```python
from build123d import *

# Parameters (mm, degrees)
SKETCH1_W                        = 39
SKETCH1_H                        = 37
BOSS_EXTRUDE1_DEPTH              = 6.5
SKETCH2_W                        = 30.2
SKETCH2_H                        = 4
CUT_EXTRUDE1_DEPTH               = 38
F_10_0_10_DIAMETER_HOLE1_D       = 10
F_10_0_10_DIAMETER_HOLE1_DEPTH   = 2.5
F_2_05_2_05_DIAMETER_HOLE1_D     = 2.05
F_2_05_2_05_DIAMETER_HOLE1_DEPTH = 6.5
F_2_05_2_05_DIAMETER_HOLE2_D     = 2.05
F_2_05_2_05_DIAMETER_HOLE2_DEPTH = 6.5
F_2_05_2_05_DIAMETER_HOLE3_D     = 2.05
F_2_05_2_05_DIAMETER_HOLE3_DEPTH = 6.5
CHAMFER1_SIZE                    = 0.25625
CHAMFER2_SIZE2                   = 0.199948225
CHAMFER2_SIZE                    = 0.199946154
SKETCH11_R                       = 1.28125
BOSS_EXTRUDE3_DEPTH              = 2.5
SKETCH12_R                       = 1.175
CUT_EXTRUDE2_DEPTH               = 7.5


with BuildPart() as part:
    # Sketch1 → Boss-Extrude1 (new body)
    with BuildSketch(Plane.XY.offset(-17)):
        with Locations((0, -3.5)):
            Rectangle(SKETCH1_W, SKETCH1_H)
    extrude(amount=-BOSS_EXTRUDE1_DEPTH)

    # Sketch2 → Cut-Extrude1 (cut, through all)
    with BuildSketch(Plane.XZ.offset(22)):
        with Locations((0, -19)):
            Rectangle(SKETCH2_W, SKETCH2_H)
    extrude(amount=-CUT_EXTRUDE1_DEPTH, mode=Mode.SUBTRACT)

    # Ø10.0 (10) Diameter Hole1
    with Locations(Plane.XY.offset(-21)):
        with Locations((0, 0)):
            Hole(F_10_0_10_DIAMETER_HOLE1_D / 2, depth=F_10_0_10_DIAMETER_HOLE1_DEPTH)

    # Ø2.05 (2.05) Diameter Hole1
    with Locations(Plane(origin=(0, 0, -23.5), x_dir=(-1, 0, 0), z_dir=(0, 0, -1))):
        with Locations((-17.3, -18), (17.3, -18), (-17.3, -11), (17.3, -11)):
            Hole(F_2_05_2_05_DIAMETER_HOLE1_D / 2, depth=F_2_05_2_05_DIAMETER_HOLE1_DEPTH)

    # Ø2.05 (2.05) Diameter Hole2
    with Locations(Plane.XY.offset(-17)):
        with Locations((17.3, 4), (-17.3, 4), (17.3, 11), (-17.3, 11)):
            Hole(F_2_05_2_05_DIAMETER_HOLE2_D / 2, depth=F_2_05_2_05_DIAMETER_HOLE2_DEPTH)

    # Ø2.05 (2.05) Diameter Hole3
    with Locations(Plane(origin=(0, 0, -23.5), x_dir=(-1, 0, 0), z_dir=(0, 0, -1))):
        with Locations((0, 11), (-7.778174593, 7.778174593), (-11, 0), (-7.778174593, -7.778174593), (0, -11), (7.778174593, -7.778174593), (11, 0), (7.778174593, 7.778174593), (13, 11), (-13, 11), (13, -17), (-13, -17)):
            Hole(F_2_05_2_05_DIAMETER_HOLE3_D / 2, depth=F_2_05_2_05_DIAMETER_HOLE3_DEPTH)

    # Chamfer1
    chamfer1_edges = [part.edges().sort_by_distance(p)[0] for p in [
        (-19.5, -3.5, -23.5),
        (-8.803174593, 7.778174593, -23.5),
        (-12.025, 0, -23.5),
        (-8.803174593, -7.778174593, -23.5),
        (-1.025, -11, -23.5),
        (6.753174593, -7.778174593, -23.5),
        (9.975, 0, -23.5),
        (6.753174593, 7.778174593, -23.5),
        (-1.025, 11, -23.5),
        (15.1, -3.5, -17),
        (-15.1, -3.5, -17),
        (-18.325, -11, -23.5),
        (-18.325, -11, -17),
        (19.5, -3.5, -23.5),
        (16.275, -11, -23.5),
        (16.275, -11, -17),
        (-18.325, -18, -23.5),
        (-18.325, -18, -17),
        (16.275, -18, -23.5),
        (16.275, -18, -17),
        (-19.5, -3.5, -17),
        (-16.275, 11, -17),
        (-16.275, 11, -23.5),
        (19.5, -3.5, -17),
        (18.325, 11, -17),
        (18.325, 11, -23.5),
        (-16.275, 4, -17),
        (-16.275, 4, -23.5),
        (18.325, 4, -17),
        (18.325, 4, -23.5),
        (11.975, -17, -23.5),
        (-14.025, -17, -23.5),
        (11.975, 11, -23.5),
        (-14.025, 11, -23.5),
    ]]
    chamfer(chamfer1_edges, length=CHAMFER1_SIZE)

    # Chamfer2
    chamfer2_edges = [part.edges().sort_by_distance(p)[0] for p in [
        (5, 0, -21),
        (5, 0, -23.5),
    ]]
    chamfer(chamfer2_edges, length=CHAMFER2_SIZE, length2=CHAMFER2_SIZE2)

    # Sketch11 → Boss-Extrude3 (add)
    with BuildSketch(Plane(origin=(0, 0, -23.5), x_dir=(-1, 0, 0), z_dir=(0, 0, -1))):
        with Locations((13, 11)):
            Circle(SKETCH11_R)
        with Locations((13, -17)):
            Circle(SKETCH11_R)
        with Locations((-13, -17)):
            Circle(SKETCH11_R)
        with Locations((-13, 11)):
            Circle(SKETCH11_R)
    extrude(amount=-BOSS_EXTRUDE3_DEPTH)

    # Sketch12 → Cut-Extrude2 (cut, through all)
    with BuildSketch(Plane.XY.offset(-17)):
        with Locations((12.7, 9)):
            Circle(SKETCH12_R)
        with Locations((-12.7, 9)):
            Circle(SKETCH12_R)
        with Locations((12.7, -16)):
            Circle(SKETCH12_R)
        with Locations((-12.7, -16)):
            Circle(SKETCH12_R)
        with Locations((-17.3, -18)):
            Circle(SKETCH12_R)
        with Locations((-17.3, -11)):
            Circle(SKETCH12_R)
        with Locations((-17.3, 4)):
            Circle(SKETCH12_R)
        with Locations((-17.3, 11)):
            Circle(SKETCH12_R)
        with Locations((17.3, -18)):
            Circle(SKETCH12_R)
        with Locations((17.3, -11)):
            Circle(SKETCH12_R)
        with Locations((17.3, 4)):
            Circle(SKETCH12_R)
        with Locations((17.3, 11)):
            Circle(SKETCH12_R)
    extrude(amount=-CUT_EXTRUDE2_DEPTH, mode=Mode.SUBTRACT)


solid = part.part
```
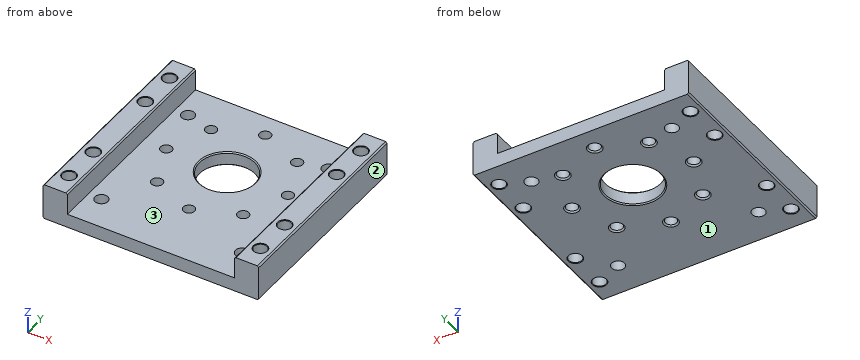
Part model, mm, in its own coordinate system. Face numbers are marked on the shaded views. Round coordinates to 2 decimals unless told otherwise and drop trailing zeros. Order: outer loops, then holes, each group sorted by start corner. A loop starts at its lowest first (then second) coordinate and runs counter-clockwise, first axis right, second up. Notation, with made-up numbers: M 12,81 L 18,81 A11 ccw 18,94 Z; hole C 37.5,51.5 d5. An arc over 180 degrees is marked long. Answer in a Markdown table with one row per item. Add a question column.
Q1. Pin check, flat tips, straight feed: pin 1 (1.4 mm diameter, centred on x = -12.7, y = -16, fed in from -Z); pin 2 (3.5 mm diameter, centred on x = -7.78, y = 7.78, fed in from +Z). Stop position of each tip, or through.
Q2. Cut at B-B on x = -11. Give the cut face in (y, z) (3 decimals), and give its area (3 significant figures).
Q3. Wall check: L1, parallel to Y at x = -12.7, z = -23 (3 decimals); L2, parallel to X at y = 0, z = -18.75; L3, parallel to Z at x = 2.5, y = 11.5. Give the ranges that are in metal, low to high. Write a range as from..to.
Q4. Cut at D-D on x = 0. Give the cut face in (y, z) (3 decimals), and give its area (3 significant figures).
Q5. Cut at A-A on z = -19. Give the number of separate pieces and of enclosed holes in the cut face, and give its area (3 significant figures).
Q6. Mould opens along X. For the marked faces 1, 2 and 3 say: +X half, -X half, draft (parallel to the pull), parting line (faces both ways), or undercut.
Established:
| question | item | result |
|---|---|---|
| 1 | pin 1 | passes through |
| 1 | pin 2 | stops at z = -21 |
| 2 | outline | M -22,-23.5 L -1.281,-23.5 L -1.025,-23.244 L -1.025,-21 L -22,-21 Z; M 1.025,-23.244 L 1.281,-23.5 L 15,-23.5 L 15,-21 L 1.025,-21 Z |
| 2 | area | 87.3 mm2 |
| 3 | L1 | y = -22..-17.175, -14.825..7.825, 10.175..15 |
| 3 | L2 | x = -19.5..-15.1, 15.1..19.5 |
| 3 | L3 | z = -23.5..-21 |
| 4 | outline | M -22,-23.5 L -12.281,-23.5 L -12.025,-23.244 L -12.025,-21 L -22,-21 Z; M -9.975,-23.244 L -9.719,-23.5 L -5.2,-23.5 L -5,-23.3 L -5,-21.2 L -5.2,-21 L -9.975,-21 Z; M 5,-23.3 L 5.2,-23.5 L 9.719,-23.5 L 9.975,-23.244 L 9.975,-21 L 5.2,-21 L 5,-21.2 Z; M 12.025,-23.244 L 12.281,-23.5 L 15,-23.5 L 15,-21 L 12.025,-21 Z |
| 4 | area | 57.0 mm2 |
| 5 | separate pieces | 2 |
| 5 | enclosed holes | 8 |
| 5 | area | 291 mm2 |
| 6 | face 1 | draft |
| 6 | face 2 | +X half |
| 6 | face 3 | undercut |
